```python
from build123d import *

# Parameters (mm, degrees)
BOSS_EXTRUDE1_DEPTH       = 10
F_6_CLEARANCE_HOLE1_D     = 3.7973
F_6_CLEARANCE_HOLE1_DEPTH = 20.001
F_6_CLEARANCE_HOLE1_TIP   = 1.140824014
F_6_CLEARANCE_HOLE2_D     = 3.7973


with BuildPart() as part:
    # Sketch1 → Boss-Extrude1 (new, symmetric)
    with BuildSketch(Plane.XY):
        Polygon((0, 20), (0, 0), (20, 0), (20, 1.5875), (1.5875, 1.5875), (1.5875, 20), align=None)
    extrude(amount=BOSS_EXTRUDE1_DEPTH, both=True)

    # #6 Clearance Hole1
    with Locations(Plane(origin=(0, 0, 0), x_dir=(-1, 0, 0), z_dir=(0, -1, 0))):
        with Locations((-10, 0)):
            Hole(F_6_CLEARANCE_HOLE1_D / 2, depth=F_6_CLEARANCE_HOLE1_DEPTH)
            with Locations((0, 0, -(F_6_CLEARANCE_HOLE1_DEPTH + F_6_CLEARANCE_HOLE1_TIP / 2))):  # 118° drill point
                Cone(0, F_6_CLEARANCE_HOLE1_D / 2, F_6_CLEARANCE_HOLE1_TIP, mode=Mode.SUBTRACT)

    # #6 Clearance Hole2 (through all)
    with Locations(Plane.ZY):
        with Locations((0, 10)):
            Hole(F_6_CLEARANCE_HOLE2_D / 2)


solid = part.part
```
Check sheet for the modelled part. Datum: model origin and axes. Units: mm. A direction names the side the tool comes from. Round coordinates to 2 decimals unless told otherwise and drop trailing zeros. Order: outer loops, then holes, each group sorted by start corner. A loop starts at its lowest first (then second) coordinate and runs counter-clockwise, first axis right, second up.
1) Section check A-A (x = 10). Record the boundary of the cut face in (y, z).
2) Mould release check, pull along Z, two halves, no side actions. Record for faces 3 (the flat face through (1, 6, -10)), 4 (the flat face through (0, 12.4, 0.1)), 5 (the cylindrical face through (0.805, 11.882, 0.247)): +Z half, -Z half, draft (parallel to the pull), parting line (faces both ways), or undercut.
3) Section check C-C (z = 0). Record the boundary of the cut face in (x, y).
4) Section check D-D (z = 7.25). Record the boundary of the cut face in (x, y).
5) Go/stop test with flat-tipped pins: pin 1 Ø8 at (y, z) = (17.5, 5.5) entering from +X; pin 2 Ø3 at (y, z) = (10, 0) entering from +X; pin 3 Ø5.5 at (x, z) = (7.5, -1.5) entering from +Y. Record where each tip stops, or that it passes through.
6) Tool access check on faces 1 (the flat face through (12.1, 0, 0.1)), 2 (the flat face through (1.588, 13, 0)). Record the directions out of +Z, -Z, +X, -X, +Y, -Y that give a thin tool (end or side, any length) a straight path to the whole face; none if there is none.
7) Scan lines: line 1 (Y direction, x = 0.7, z = 0); line 2 (Z direction, x = 10, y = 0.8); line 3 (X direction, y = 3.5, z = 6.5). Record each from-to range of solid material in increasing order.
Result:
1. outline: (0, -10) - (1.59, -10) - (1.59, -1.9) - (0, -1.9) - close; (0, 1.9) - (1.59, 1.9) - (1.59, 10) - (0, 10) - close
2. face 3: -Z half
2. face 4: draft
2. face 5: undercut
3. outline: (0, 0) - (8.1, 0) - (8.1, 1.59) - (1.59, 1.59) - (1.59, 8.1) - (0, 8.1) - close; (0, 11.9) - (1.59, 11.9) - (1.59, 20) - (0, 20) - close; (11.9, 0) - (20, 0) - (20, 1.59) - (11.9, 1.59) - close
4. outline: (0, 0) - (20, 0) - (20, 1.59) - (1.59, 1.59) - (1.59, 20) - (0, 20) - close
5. pin 1: stops at x = 1.59
5. pin 2: passes through
5. pin 3: stops at y = 1.59
6. face 1: +Z, -Z, +X, -X, -Y
6. face 2: +Z, -Z, +X, +Y
7. line 1: y = 0 to 8.1, 11.9 to 20
7. line 2: z = -10 to -1.9, 1.9 to 10
7. line 3: x = 0 to 1.59
